Input: part model. Units: mm. Frame: model coordinates. Round coordinates to 2 decimals unless told otherwise and drop trailing zeros. Loops run counter-clockwise (first coordinate to the right, second up) from the corner with the lowest first, then second, coordinate; pieces in that order, holes last. Notation, with made-up numbers: (25.5, 4) -> (78.5, 4) arc R7 ccw to (78.5, 12) -> close; hole circle Ø1 at (80.25, -14.5). An arc over 180 degrees is marked (long way). One line per question, with ' | ' between items. Start each with the question number.
Q1. Material intervals for L1, parallel to X at y = 0.75, z = -100; L2, parallel to Z at x = 185, y = 1.7; L3, parallel to Z at x = 157, y = 0.7, sorted ascending.
Q2. Cut plane D-D on x = 12. Return loops of the section in (y, z).
Q3. Cut plane A-A on x = 83.5. Return loops of the section in (y, z), and give its area (3 significant figures).
Q4. Mould query, pull axis Z, two halves, no side actions, for faces 1 (the face through (183.34, 1.48, -0.37)), 2 (the face through (48, 3, -26)). Classes: pulls with the +Z half, pulls with the -Z half, needs draft (parallel to the pull), parting line crosses it, or undercut.
Q5. Cut plane B-B on z = -28.5. State how many separate pieces and enclosed holes the cut face has, and give its area (3 significant figures).
from build123d import *

# Parameters (mm, degrees)
SKETCH_1_W      = 195
SKETCH_1_H      = 110
SKETCH_1_R      = 1.65
SKETCH_1_R_2    = 1.7
EXTRUDE_1_DEPTH = 3


with BuildPart() as part:
    # 草图1 → 凸台-拉伸1 (new body)
    with BuildSketch(Plane(origin=(0, 0, 0), x_dir=(1, 0, 0), z_dir=(0, 1, 0))):
        with Locations((92.5, 50)):
            Rectangle(SKETCH_1_W, SKETCH_1_H)
        with Locations(Location((0, 0, 0), (0, 0, 270))):
            Circle(SKETCH_1_R, mode=Mode.SUBTRACT)
        with Locations(Location((0, 100, 0), (0, 0, 270))):
            Circle(SKETCH_1_R, mode=Mode.SUBTRACT)
        with Locations(Location((185, 100, 0), (0, 0, 270))):
            Circle(SKETCH_1_R_2, mode=Mode.SUBTRACT)
        with Locations(Location((185, 0, 0), (0, 0, 270))):
            Circle(SKETCH_1_R_2, mode=Mode.SUBTRACT)
        with BuildLine():
            Line((67.5, 6.65), (67.5, 93.35))
            ThreePointArc((67.5, 93.35), (69.15, 95), (70.8, 93.35))
            Line((70.8, 93.35), (70.8, 6.65))
            ThreePointArc((70.8, 6.65), (69.15, 5), (67.5, 6.65))
        make_face(mode=Mode.SUBTRACT)
        Polygon((5, 90), (27.352941176, 50), (5, 10), align=None, mode=Mode.SUBTRACT)
        Polygon((10, 95), (52.5, 95), (31.25, 56.973684211), align=None, mode=Mode.SUBTRACT)
        Polygon((10, 5), (52.5, 5), (31.25, 43.026315789), align=None, mode=Mode.SUBTRACT)
        Polygon((57.5, 90), (57.5, 10), (35.147058824, 50), align=None, mode=Mode.SUBTRACT)
        Polygon((85.8, 5), (175, 5), (130.4, 45.244161359), align=None, mode=Mode.SUBTRACT)
        Polygon((80.8, 10), (80.8, 90), (125.129411765, 50), align=None, mode=Mode.SUBTRACT)
        Polygon((85.8, 95), (175, 95), (130.4, 54.755838641), align=None, mode=Mode.SUBTRACT)
        Polygon((180, 10), (180, 90), (135.670588235, 50), align=None, mode=Mode.SUBTRACT)
    extrude(amount=EXTRUDE_1_DEPTH)


solid = part.part
Results:
1) L1: -5 to -1.65, 1.65 to 183.3, 186.7 to 190 | L2: -105 to -101.7, -98.3 to -1.7, 1.7 to 5 | L3: -105 to -95, -78.76 to -69.25, -30.75 to -21.24, -5 to 5
2) outline: (0, -105) -> (3, -105) -> (3, -95) -> (0, -95) -> close; (0, -91.42) -> (3, -91.42) -> (3, -77.47) -> (0, -77.47) -> close; (0, -22.53) -> (3, -22.53) -> (3, -8.58) -> (0, -8.58) -> close; (0, -5) -> (3, -5) -> (3, 5) -> (0, 5) -> close
3) outline: (0, -105) -> (3, -105) -> (3, -87.56) -> (0, -87.56) -> close; (0, -12.44) -> (3, -12.44) -> (3, 5) -> (0, 5) -> close | area: 105 mm^2
4) face 1: undercut | face 2: needs draft
5) separate pieces: 8 | enclosed holes: 0 | area: 230 mm^2
